Build history of the part. All positions in model axes, mm. A direction names the side the tool comes from. Give positions to 0.01 mm unless a question says otherwise; leave off trailing zeros. Write each loop counter-clockwise with the first axis right and the second up, starting at its lowest first coordinate (ties: lowest second). Pieces come first, ordered by that corner, then holes. Notation, with made-up numbers: (47.5, 59.25) -> (62.5, 59.25) arc R22 cw to (62.5, 86.25) -> close; hole circle Ø11 at (88, 62). An arc over 180 degrees is marked (long way). Write item = value, one per line. Start each with the question number.
Q1. Saw through at B-B, the plane z = -2.5. List the corners of the cut face in (x, y).
Q2. Wall check: line 1 (X direction, y = -7, z = 22); line 2 (Z direction, x = -31.5, y = -15); line 3 (Y direction, x = 3, z = -10.5). Give the ranges that are in metal, low to high.
Q3. Drop flat-ended pins along their axis: P1, Ø4, axis at x = 7, z = 11.5, coming from the -Y side; P2, Ø12, axis at x = -13.5, z = -11, coming from the +Y side; P3, Ø2, axis at x = -33.5, z = -19, coming from the +Y side. Give the stop position or say it passes through.
Q4. Saw through at D-D, the plane x = 39.5. List the corners of the cut face in (y, z), then the cut area to 3 significant figures.
Q5. Tool access for faces 1 (the face through (-39, -30.988, 12)), 2 (the face through (-28.723, -27.979, -8.393)), 3 (the face through (-34.586, -28.155, 19.163)): list every direction of +Z, -Z, +X, -X, +Y, -Y with a clear straight run to the whole face (end or side of a thin tool).
Q6. Mould opens along Z. For faces 4 (the face through (24, -30.988, 10)), 5 (the face through (31.64, -28.15, 6.86)) say: pulls with the +Z half, pulls with the -Z half, needs draft (parallel to the pull), parting line crosses it, or undercut.
Q7. Saw through at C-C, the plane y = -6. List the corners of the cut face in (x, z).
Q8. Saw through at A-A, the plane y = -27. Give the number of separate pieces and of enclosed holes in the cut face, then the cut area to 3 significant figures.
from build123d import *
from build123d import SkipClean  # not in build123d's __all__

# Parameters (mm, degrees)
F0_W         = 99.8685993254
F0_H         = 53.244067356
F1_DEPTH     = 25.4
F2_R         = 8.3909074383
F3_DEPTH     = 5.588
F4_T         = 0.254
F4_T6_ANGLE  = 90.000000253
F4_T8_ANGLE  = 269.999999749
F4_T12_ANGLE = 180.000000001
F4_T14_ANGLE = 180.000000001


# Not quite as in the source:
# - a shell that OpenCascade refuses in one call is made with other operations: the cavity is built on its own and cut out


with BuildPart() as f1:
    # F0 (on Front) → F1 (new body)
    with BuildSketch(Plane.XZ):
        with Locations((2.4463478476, -0.7195146754)):
            Rectangle(F0_W, F0_H)
    extrude(amount=F1_DEPTH)

    # F2 (on face) → F3 (join)
    with BuildSketch(Plane.XZ.offset(25.4)):
        with Locations((-5.1805051044, 8.3909074383)):
            Circle(F2_R)
        with Locations((23.8878745586, 10.0732017308)):
            Circle(F2_R)
        with Locations((23.600069806, -15.5415115878)):
            Circle(F2_R)
        with Locations((-4.6048937365, -18.9506409151)):
            Circle(F2_R)
        with Locations((-33.0976620317, -15.2537049726)):
            Circle(F2_R)
        with Locations((-39.0970443768, 12.0878415182)):
            Circle(F2_R)
    extrude(amount=F3_DEPTH)

    # F4: shell of thickness 0.254, made by hand


with BuildPart() as f4_core1:
    # F4_t2: copy of F1
    add(f1.part, clean=False)

    # the walls: a layer under each face that stays
    f4_faces = [f4_core1.faces().sort_by_distance(p)[0] for p in [
        (-47.4879518151, -12.7, -0.7195146754),
        (2.4463478476, -12.7, 25.9025190026),
        (2.4463478476, -12.7, -27.3415483534),
        (2.4463478476, -25.4, -0.7195146754),
        (52.3806475103, -12.7, -0.7195146754),
        (-41.48856947, -28.194, -15.2537049726),
        (-12.9958011749, -28.194, -18.9506409151),
        (15.2091623677, -28.194, -15.5415115878),
        (-47.4879518151, -28.194, 12.0878415182),
        (-13.5714125427, -28.194, 8.3909074383),
        (15.4969671202, -28.194, 10.0732017308),
        (-33.0976620317, -30.988, -15.2537049726),
        (-4.6048937365, -30.988, -18.9506409151),
        (23.600069806, -30.988, -15.5415115878),
        (-39.0970443768, -30.988, 12.0878415182),
        (-5.1805051044, -30.988, 8.3909074383),
        (23.8878745586, -30.988, 10.0732017308),
    ]]
    thicken(f4_faces, amount=-F4_T, mode=Mode.SUBTRACT)

    # F4_s3 → F4_t4 (revolve, cut)
    with BuildSketch(Plane.XY.offset(-15.2537049726)):
        Polygon((-24.7042145933, -25.40254), (-24.7067545933, -25.146), (-24.9607545933, -25.146), (-24.9607545933, -25.4), align=None)
    revolve(axis=Axis((-33.0976620317, -25.4, -15.2537049726), (0, -1, 0)), mode=Mode.SUBTRACT)

    # F4_s5 → F4_t6 (revolve, cut)
    with BuildSketch(Plane.YZ.offset(-4.6048937365)):
        Polygon((-25.40254, -27.3440883534), (-25.146, -27.3415483534), (-25.146, -27.0875483534), (-25.4, -27.0875483534), align=None)
    revolve(axis=Axis((-4.6048937365, -25.4, -18.9506409151), (0, -1, 0)), revolution_arc=F4_T6_ANGLE, mode=Mode.SUBTRACT)

    # F4_s7 → F4_t8 (revolve, cut)
    with BuildSketch(Plane.XY.offset(-18.9506409151)):
        Polygon((3.7885537018, -25.40254), (3.7860137018, -25.146), (3.5320137018, -25.146), (3.5320137018, -25.4), align=None)
    revolve(axis=Axis((-4.6048937365, -25.4, -18.9506409151), (0, -1, 0)), revolution_arc=F4_T8_ANGLE, mode=Mode.SUBTRACT)

    # F4_s9 → F4_t10 (revolve, cut)
    with BuildSketch(Plane.XY.offset(-15.5415115878)):
        Polygon((31.9935172443, -25.40254), (31.9909772443, -25.146), (31.7369772443, -25.146), (31.7369772443, -25.4), align=None)
    revolve(axis=Axis((23.600069806, -25.4, -15.5415115878), (0, -1, 0)), mode=Mode.SUBTRACT)

    # F4_s11 → F4_t12 (revolve, cut)
    with BuildSketch(Plane.XY.offset(12.0878415182)):
        Polygon((-47.4904918151, -25.40254), (-47.4879518151, -25.146), (-47.2339518151, -25.146), (-47.2339518151, -25.4), align=None)
    with SkipClean():  # cleaning this boolean's faces spoils the solid; the shape is the same uncleaned
        revolve(axis=Axis((-39.0970443768, -25.4, 12.0878415182), (0, -1, 0)), revolution_arc=F4_T12_ANGLE, mode=Mode.SUBTRACT)

    # F4_s13 → F4_t14 (revolve, cut)
    with BuildSketch(Plane.XY.offset(12.0878415182)):
        Polygon((-30.7035969385, -25.40254), (-30.7061369385, -25.146), (-30.9601369385, -25.146), (-30.9601369385, -25.4), align=None)
    revolve(axis=Axis((-39.0970443768, -25.4, 12.0878415182), (0, -1, 0)), revolution_arc=F4_T14_ANGLE, mode=Mode.SUBTRACT)

    # F4_s15 → F4_t16 (revolve, cut)
    with BuildSketch(Plane.XY.offset(8.3909074383)):
        Polygon((3.212942334, -25.40254), (3.210402334, -25.146), (2.956402334, -25.146), (2.956402334, -25.4), align=None)
    revolve(axis=Axis((-5.1805051044, -25.4, 8.3909074383), (0, -1, 0)), mode=Mode.SUBTRACT)

    # F4_s17 → F4_t18 (revolve, cut)
    with BuildSketch(Plane.XY.offset(10.0732017308)):
        Polygon((32.2813219969, -25.40254), (32.2787819969, -25.146), (32.0247819969, -25.146), (32.0247819969, -25.4), align=None)
    revolve(axis=Axis((23.8878745586, -25.4, 10.0732017308), (0, -1, 0)), mode=Mode.SUBTRACT)


with BuildPart() as f1_1:
    add(f1.part, clean=False)

    # what is left inside the walls is the cavity
    f4_cavity = [f4_core1.part.solids().sort_by_distance(p)[0] for p in [
        (2.446348, -0.00254, -9.508859),
    ]]
    add(f4_cavity, mode=Mode.SUBTRACT)


solid = f1_1.part
Report:
q1.outline = (-47.49, -25.4) -> (52.38, -25.4) -> (52.38, 0) -> (52.13, 0) -> (52.13, -25.15) -> (-47.23, -25.15) -> (-47.23, 0) -> (-47.49, 0) -> close
q2.line_1 = -47.49 to -47.23, 52.13 to 52.38
q2.line_2 = -27.34 to -27.09, 25.65 to 25.9
q2.line_3 = -25.4 to -25.15
q3.P1 = -25.4
q3.P2 = -25.15
q3.P3 = -30.73
q4.outline = (-25.4, -27.34) -> (0, -27.34) -> (0, -27.09) -> (-25.15, -27.09) -> (-25.15, 25.65) -> (0, 25.65) -> (0, 25.9) -> (-25.4, 25.9) -> close
q4.area = 26.3 mm2
q5.face_1 = +Z, -Z, +X, -X, -Y
q5.face_2 = +Y
q5.face_3 = -Y
q6.face_4 = needs draft
q6.face_5 = undercut
q7.outline = (-47.49, -27.34) -> (52.38, -27.34) -> (52.38, 25.9) -> (-47.49, 25.9) -> close; hole (-47.23, -27.09) -> (52.13, -27.09) -> (52.13, 25.65) -> (-47.23, 25.65) -> close
q8.separate_pieces = 6
q8.enclosed_holes = 6
q8.area = 79.1 mm2
